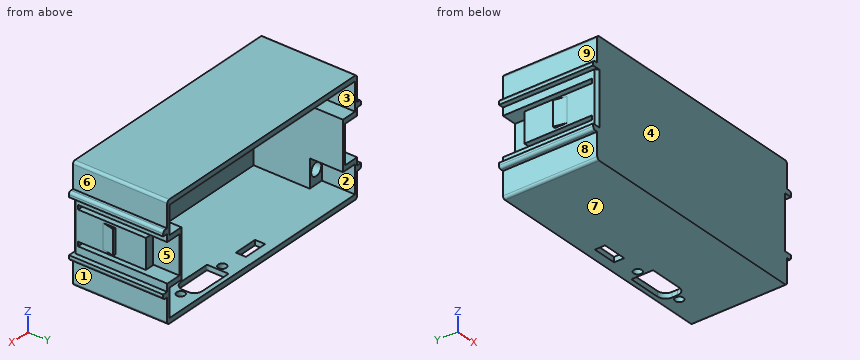
```python
from build123d import *

# Parameters (mm, degrees)
SKETCH1_W            = 47
SKETCH1_H            = 45
BOSS_EXTRUDE1_DEPTH  = 2
BOSS_EXTRUDE3_DEPTH  = 35
BOSS_EXTRUDE4_DEPTH  = 4.8
SKETCH6_W            = 2
SKETCH6_H            = 2
BOSS_EXTRUDE5_DEPTH  = 37
SKETCH13_W           = 6
SKETCH13_H           = 11
BOSS_EXTRUDE7_DEPTH  = 22
SKETCH23_W           = 3.5
SKETCH23_H           = 26.6
BOSS_EXTRUDE9_DEPTH  = 1
SKETCH24_W           = 3.5
SKETCH24_H           = 26.6
BOSS_EXTRUDE10_DEPTH = 1
HOLE2_D              = 3.2
HOLE2_DEPTH          = 15
HOLE2_CBORE_D        = 5
HOLE2_CBORE_DEPTH    = 5
FILLET1_R            = 1
FILLET2_R            = 1
SKETCH25_W           = 1
SKETCH25_H           = 15
CUT_EXTRUDE5_DEPTH   = 35
FILLET1_OF_MIRROR1_R = 1
FILLET2_OF_MIRROR1_R = 1
CHAMFER1_SIZE        = 1
SKETCH19_R           = 1.6
CUT_EXTRUDE1_DEPTH   = 10
SKETCH20_W           = 9.5
SKETCH20_H           = 4
CUT_EXTRUDE2_DEPTH   = 10


with BuildPart() as part:
    # Sketch1 → Boss-Extrude1 (new body)
    with BuildSketch(Plane(origin=(0, 0, 0), x_dir=(1, 0, 0), z_dir=(0, 1, 0))):
        with Locations((-23.5, 22.5)):
            Rectangle(SKETCH1_W, SKETCH1_H)
    boss_extrude1 = extrude(amount=BOSS_EXTRUDE1_DEPTH)

    # Sketch4 → Boss-Extrude3 (add)
    with BuildSketch(Plane(origin=(0, 2, 0), x_dir=(1, 0, 0), z_dir=(0, 1, 0))):
        Polygon((-42, 15), (-47, 15), (-47, 0), (0, 0), (0, 2), (-0.864229009, 2), (-2, 2), (-45, 2), (-46, 2), (-46, 13), (-45, 13), (-40, 13), (-40, 32), (-45, 32), (-46, 32), (-46, 43), (-45, 43), (-2, 43), (0, 43), (0, 45), (-47, 45), (-47, 30), (-42, 30), align=None)
    boss_extrude3 = extrude(amount=BOSS_EXTRUDE3_DEPTH)

    # Sketch5 → Boss-Extrude4 (add, symmetric)
    with BuildSketch(Plane.XY.offset(-22.5)):
        Polygon((-47, 2), (-47, 11.8), (-48, 16.6), (-47, 16.6), (-47, 28.6), (-43.5, 28.6), (-43.5, 2), align=None)
    boss_extrude4 = extrude(amount=BOSS_EXTRUDE4_DEPTH, both=True)

    # Sketch6 → Boss-Extrude5 (add)
    with BuildSketch(Plane(origin=(0, 0, 0), x_dir=(-1, 0, 0), z_dir=(0, -1, 0))):
        with Locations((48, 34)):
            Rectangle(SKETCH6_W, SKETCH6_H)
        with Locations((48, 11)):
            Rectangle(SKETCH6_W, SKETCH6_H)
    boss_extrude5 = extrude(amount=-BOSS_EXTRUDE5_DEPTH)

    # Sketch13 → Boss-Extrude7 (add)
    with BuildSketch(Plane(origin=(0, 2, 0), x_dir=(1, 0, 0), z_dir=(0, 1, 0))):
        with Locations((-43, 37.5)):
            Rectangle(SKETCH13_W, SKETCH13_H)
        with Locations((-43, 7.5)):
            Rectangle(SKETCH13_W, SKETCH13_H)
    boss_extrude7 = extrude(amount=BOSS_EXTRUDE7_DEPTH)

    # Sketch23 → Boss-Extrude9 (add)
    with BuildSketch(Plane.XY.offset(-17.7)):
        with Locations((-45.25, 15.3)):
            Rectangle(SKETCH23_W, SKETCH23_H)
    boss_extrude9 = extrude(amount=BOSS_EXTRUDE9_DEPTH)

    # Sketch24 → Boss-Extrude10 (add)
    with BuildSketch(Plane(origin=(0, 0, -27.3), x_dir=(-1, 0, 0), z_dir=(0, 0, -1))):
        with Locations((45.25, 15.3)):
            Rectangle(SKETCH24_W, SKETCH24_H)
    boss_extrude10 = extrude(amount=BOSS_EXTRUDE10_DEPTH)

    # Hole2
    with Locations(Plane(origin=(-43.2, 24, -7.5), x_dir=(0, 0, 1), z_dir=(0, 1, 0))):
        with Locations((0, 0), (-30, 0)):
            hole2 = CounterBoreHole(HOLE2_D / 2, HOLE2_CBORE_D / 2, HOLE2_CBORE_DEPTH, depth=HOLE2_DEPTH)

    # Fillet1
    fillet1_edges = [part.edges().sort_by_distance(p)[0] for p in [
        (-47, 18.5, 0),
        (-47, 18.5, -45),
        (-49, 18.5, -35),
        (-49, 18.5, -10),
    ]]
    fillet(fillet1_edges, radius=FILLET1_R)

    # Fillet2
    fillet2_edges = [part.edges().sort_by_distance(p)[0] for p in [
        (-43.5, 2, -22.5),
    ]]
    fillet(fillet2_edges, radius=FILLET2_R)

    # Sketch25 → Cut-Extrude5 (cut)
    with BuildSketch(Plane(origin=(0, 37, 0), x_dir=(1, 0, 0), z_dir=(0, 1, 0))):
        with Locations((-41.5, 22.5)):
            Rectangle(SKETCH25_W, SKETCH25_H)
    cut_extrude5 = extrude(amount=-CUT_EXTRUDE5_DEPTH, mode=Mode.SUBTRACT)

    # Mirror1: Boss-Extrude1, Boss-Extrude3, Boss-Extrude4, Boss-Extrude5, Boss-Extrude7, Boss-Extrude9, Boss-Extrude10, Hole2, Cut-Extrude5 across plane
    add(boss_extrude1.mirror(Plane(origin=(0, 0, 0), x_dir=(0, 0, 1), z_dir=(1, 0, 0))))
    add(boss_extrude3.mirror(Plane(origin=(0, 0, 0), x_dir=(0, 0, 1), z_dir=(1, 0, 0))))
    add(boss_extrude4.mirror(Plane(origin=(0, 0, 0), x_dir=(0, 0, 1), z_dir=(1, 0, 0))))
    add(boss_extrude5.mirror(Plane(origin=(0, 0, 0), x_dir=(0, 0, 1), z_dir=(1, 0, 0))))
    add(boss_extrude7.mirror(Plane(origin=(0, 0, 0), x_dir=(0, 0, 1), z_dir=(1, 0, 0))))
    add(boss_extrude9.mirror(Plane(origin=(0, 0, 0), x_dir=(0, 0, 1), z_dir=(1, 0, 0))))
    add(boss_extrude10.mirror(Plane(origin=(0, 0, 0), x_dir=(0, 0, 1), z_dir=(1, 0, 0))))
    add(hole2.mirror(Plane(origin=(0, 0, 0), x_dir=(0, 0, 1), z_dir=(1, 0, 0))), mode=Mode.SUBTRACT)
    add(cut_extrude5.mirror(Plane(origin=(0, 0, 0), x_dir=(0, 0, 1), z_dir=(1, 0, 0))), mode=Mode.SUBTRACT)

    # Fillet1 of Mirror1
    fillet1_of_mirror1_edges = [part.edges().sort_by_distance(p)[0] for p in [
        (47, 18.5, 0),
        (47, 18.5, -45),
        (49, 18.5, -35),
        (49, 18.5, -10),
    ]]
    fillet(fillet1_of_mirror1_edges, radius=FILLET1_OF_MIRROR1_R)

    # Fillet2 of Mirror1
    fillet2_of_mirror1_edges = [part.edges().sort_by_distance(p)[0] for p in [
        (43.5, 2, -22.5),
    ]]
    fillet(fillet2_of_mirror1_edges, radius=FILLET2_OF_MIRROR1_R)

    # Chamfer1
    chamfer1_edges = [part.edges().sort_by_distance(p)[0] for p in [
        (47, 0, -22.5),
        (-47, 0, -22.5),
    ]]
    chamfer(chamfer1_edges, length=CHAMFER1_SIZE)

    # Sketch19 → Cut-Extrude1 (cut)
    with BuildSketch(Plane(origin=(-58.916405474, -6.932652766, -45), x_dir=(-1, 0, 0), z_dir=(0, 0, -1))):
        with Locations((-91.616405474, 37.882652766)):
            Circle(SKETCH19_R)
        with Locations((-71.016405474, 37.882652766)):
            Circle(SKETCH19_R)
        with BuildLine():
            Line((-73.666405474, 42.132652766), (-86.166405474, 42.132652766))
            ThreePointArc((-86.166405474, 42.132652766), (-88.429147174, 41.195394466), (-89.366405474, 38.932652766))
            Line((-89.366405474, 38.932652766), (-89.366405474, 36.832652766))
            ThreePointArc((-89.366405474, 36.832652766), (-88.429147174, 34.569911067), (-86.166405474, 33.632652766))
            Line((-86.166405474, 33.632652766), (-73.666405474, 33.632652766))
            ThreePointArc((-73.666405474, 33.632652766), (-73.383562762, 33.749810054), (-73.266405474, 34.032652766))
            Line((-73.266405474, 34.032652766), (-73.266405474, 41.732652766))
            ThreePointArc((-73.266405474, 41.732652766), (-73.383562762, 42.015495479), (-73.666405474, 42.132652766))
        make_face()
    extrude(amount=-CUT_EXTRUDE1_DEPTH, mode=Mode.SUBTRACT)

    # Sketch20 → Cut-Extrude2 (cut)
    with BuildSketch(Plane(origin=(-58.916405474, -6.932652766, -45), x_dir=(-1, 0, 0), z_dir=(0, 0, -1))):
        with Locations((-57.496405474, 38.232652766)):
            Rectangle(SKETCH20_W, SKETCH20_H)
    extrude(amount=-CUT_EXTRUDE2_DEPTH, mode=Mode.SUBTRACT)


solid = part.part
```
Here's how the part is built. I have some questions about the finished solid (model axes, mm). Face numbers are marked on the shaded views. A direction names the side the tool comes from. Coordinates: 2 decimals unless noted, no trailing zeros. Order: outer loops, then holes, each group sorted by start corner. A loop starts at its lowest first (then second) coordinate and runs counter-clockwise, first axis right, second up.
Item 1: If we section it at D-D, the plane x = -33: List the corners of the cut face in (y, z) for me, then the cut area to 3 significant figures.
Response values:
outline: (0, -45) - (37, -45) - (37, -43) - (2, -43) - (2, -2) - (37, -2) - (37, 0) - (0, 0) - close
area: 230 mm2
Item 2: If we section it at A-A, the plane x = 12.1: List the corners of the cut face in (y, z) for me, then the cut area to 3 significant figures.
Response values:
outline: (0, -45) - (29.35, -45) - (29.35, -43) - (2, -43) - (2, -2) - (37, -2) - (37, 0) - (0, 0) - close; (32.55, -45) - (37, -45) - (37, -43) - (32.55, -43) - close
area: 224 mm2
Item 3: Which directions (+Z, -Z, +X, -X, +Y, -Y) give clear straight access to the entire face, cutting with the end or side of a thin tool? Please do the marked faces 5, 6, 7, 8 and 9.
Response values:
face 5: +Y
face 6: +Z, +X, +Y, -Y
face 7: -Z, +X, -X, +Y, -Y
face 8: -Z, -X, +Y, -Y
face 9: +Z, -X, +Y, -Y
Item 4: Thinking about a two-plate mould opening in X: for the marked faces 1, 2, 3 and 4, which applies, pulls with the +X half, pulls with the -X half, needs draft (parallel to the pull), parting line crosses it, or undercut?
Response values:
face 1: pulls with the +X half
face 2: undercut
face 3: undercut
face 4: needs draft
Item 5: I'm going to push flat-ended pins straight in: pin 1 Ø2 at (x, z) = (20.5, -29.5) entering from +Y; pin 2 Ø8 at (x, z) = (22.5, -7) entering from -Y; pin 3 Ø3.5 at (y, z) = (31.5, -8.5) entering from +X; pin 4 Ø1.5 at (x, y) = (47.5, 27) entering from -Z. Where does each tip first touch, or does it pass through?
Response values:
pin 1: stops at y = 2
pin 2: stops at y = 0
pin 3: stops at x = 48.66
pin 4: stops at z = -44.66
Item 6: I need wall thicknesses on probe 1 along X at (y, z) = (20, -7.5); probe 2 along Z at (x, y) = (43.2, 11.5); probe 3 along Z at (x, y) = (4.5, 18.5). Which ranges of each line are inside material? Lowest first, please.
Response values:
probe 1: x = -47 to -45.7, -40.7 to -40, 40 to 40.7, 45.7 to 47
probe 2: z = -45 to -39.1, -35.9 to -30, -15 to -9.1, -5.9 to 0
probe 3: z = -45 to -43, -2 to 0
Item 7: If we section it at C-C, the plane y = 7.5: Give the number of separate pieces and of enclosed holes in the cut face, then the cut area to 3 significant figures.
Response values:
separate pieces: 3
enclosed holes: 1
area: 865 mm2
Item 8: If we section it at B-B, the plane z = -31: List the corners of the cut face in (x, y) for me, then the cut area to 3 significant figures.
Response values:
outline: (-47, 1) - (-46, 0) - (46, 0) - (47, 1) - (47, 37) - (40, 37) - (40, 2) - (-40, 2) - (-40, 37) - (-47, 37) - close
area: 677 mm2
